```python
from build123d import *

# Parameters (mm, degrees)
F1_DEPTH = 25.4
F2_T     = -2.54
F3_R     = 2.754178
F3_R_2   = 3.516822
F4_DEPTH = 59.182


with BuildPart() as f1:
    # F0 (on Front) → F1 (new body)
    with BuildSketch(Plane.XZ):
        with BuildLine():
            Line((-66.046305, 23.096353), (-66.046305, 6.816403))
            Line((-66.046305, 6.816403), (-17.603524, 6.816403))
            Line((-17.603524, 6.816403), (-17.603524, 20.350474))
            ThreePointArc((-17.603524, 20.350474), (-18.407773, 22.292103), (-20.349403, 23.096353))
            Line((-20.349403, 23.096353), (-64.987443, 23.096353))
            Line((-64.987443, 23.096353), (-66.046305, 23.096353))
        make_face()
    extrude(amount=F1_DEPTH)

    # F2
    f2_openings = [f1.faces().sort_by_distance(p)[0] for p in [
        (-43.197854, -12.7, 23.096353),
        (-17.603524, -12.7, 13.583438),
        (-18.407773, -12.7, 22.292103),
        (-66.046305, -12.7, 14.956378),
    ]]
    offset(amount=F2_T, openings=f2_openings)

    # F3 (on Front) + F1_face (on face) → F4 (cut)
    with BuildSketch(Plane.XZ):
        with Locations((-27.133251, 14.36077)):
            Circle(F3_R)
        with Locations((-52.810572, 15.287271)):
            Circle(F3_R_2)
    with BuildSketch(Plane(origin=(-41.873451, -25.4, 14.940904), x_dir=(1, 0, 0), z_dir=(0, -1, 0))):
        with BuildLine():
            Line((-24.172854, 8.155449), (-24.172854, -8.124501))
            Line((-24.172854, -8.124501), (24.269927, -8.124501))
            Line((24.269927, -8.124501), (24.269927, 5.40957))
            ThreePointArc((24.269927, 5.40957), (23.465677, 7.3512), (21.524048, 8.155449))
            Line((21.524048, 8.155449), (-24.172854, 8.155449))
        make_face()
    extrude(amount=F4_DEPTH, mode=Mode.SUBTRACT)


solid = f1.part
```
The listing builds one solid part. Answer for the finished solid, in the listing's coordinates (mm). A direction names the side the tool comes from. Give positions to 0.01 mm unless a question says otherwise; leave off trailing zeros. Loops run counter-clockwise (first coordinate to the right, second up) from the corner with the lowest first, then second, coordinate; pieces in that order, holes last. Notation, with made-up numbers: (83, -12) - (104, -12) arc R12 cw to (104, 9) - close; hole circle Ø1 at (75.5, 30). An arc over 180 degrees is marked (long way). Answer as CSV lines item,"result". Start each with the question number.
Item 1: For faces 4 (the face through (-56.324, -1.252, 15.442)), 5 (the face through (-42, -13, 9.356)), determine the directions among +Z, -Z, +X, -X, +Y, -Y from which every point of the face is accessible in a straight line to the end or side of a thin tool.
Item 2: A cutting plane is placed at C-C on z = 13. Determine the outline of the cut face in (x, y).
Item 3: Each of these flat-tipped pins is pushed along its axis until it touches: pin 1 (6 mm diameter, centred on y = -6, z = 21, fed in from +X); pin 2 (3 mm diameter, centred on x = -45.5, y = -8, fed in from +Z). Where does it stop, or does it pass through?
Item 4: A cutting plane is placed at A-A on z = 11. Determine the outline of the cut face in (x, y).
Item 5: A cutting plane is placed at B-B on x = -34.5. Determine the outline of the cut face in (y, z).
Item 6: Find the intervals of material crossed by line 1 (Y direction, x = -27, z = 10.5); line 2 (X direction, y = -2.5, z = 16.5); line 3 (Z direction, x = -49.5, y = -6), in increasing order. Write a range as from..to.
Item 7: A cutting plane is placed at D-D on y = -16.5. Determine the outline of the cut face in (x, z).
Item 8: The mould has two halves that part along Y. Classify faces 1 (the face through (-27.73, -24.11, 11.67)), 2 (the face through (-42, -2.54, 16)), 3 (the face through (-42, -25.4, 15)): +Y half, -Y half, draft (parallel to the pull), parting line (faces both ways), or undercut.
Found:
1,face 4,"+Y, -Y"
1,face 5,"+Z, +X, -X"
2,outline,"(-66.05, -25.4) - (-55.48, -25.4) - (-55.48, -22.86) - (-66.05, -22.86) - close; (-66.05, -2.54) - (-55.48, -2.54) - (-55.48, 0) - (-66.05, 0) - close; (-50.14, -25.4) - (-29.53, -25.4) - (-29.53, -22.86) - (-50.14, -22.86) - close; (-50.14, -2.54) - (-29.53, -2.54) - (-29.53, 0) - (-50.14, 0) - close; (-24.74, -25.4) - (-17.6, -25.4) - (-17.6, -22.86) - (-24.74, -22.86) - close; (-24.74, -2.54) - (-17.6, -2.54) - (-17.6, 0) - (-24.74, 0) - close"
3,pin 1,"passes through"
3,pin 2,"stops at z = 9.36"
4,outline,"(-66.05, -25.4) - (-17.6, -25.4) - (-17.6, -22.86) - (-66.05, -22.86) - close; (-66.05, -2.54) - (-17.6, -2.54) - (-17.6, 0) - (-66.05, 0) - close"
5,outline,"(-25.4, 6.82) - (0, 6.82) - (0, 23.1) - (-2.54, 23.1) - (-2.54, 9.36) - (-22.86, 9.36) - (-22.86, 23.1) - (-25.4, 23.1) - close"
6,line 1,"y = -25.4..-22.86, -2.54..0"
6,line 2,"x = -66.05..-56.11, -49.51..-28.87, -25.4..-17.6"
6,line 3,"z = 6.82..9.36"
7,outline,"(-66.05, 6.82) - (-17.6, 6.82) - (-17.6, 9.36) - (-66.05, 9.36) - close"
8,face 1,"draft"
8,face 2,"undercut"
8,face 3,"-Y half"
